```python
from build123d import *

# Parameters (mm, degrees)
F0_R     = 2.5
F1_DEPTH = 300


with BuildPart() as f1:
    # F0 (on Top) → F1 (new body)
    with BuildSketch(Plane.XY):
        with BuildLine():
            ThreePointArc((-10.36, 12.5), (-11.873209, 11.873209), (-12.5, 10.36))
            Line((-12.5, 10.36), (-12.5, 4.32))
            ThreePointArc((-12.5, 4.32), (-11.43, 3.25), (-10.36, 4.32))
            Line((-10.36, 4.32), (-10.36, 6.263583))
            ThreePointArc((-10.36, 6.263583), (-9.699471, 7.252134), (-8.533396, 7.020187))
            Line((-8.533396, 7.020187), (-4.363396, 2.850187))
            ThreePointArc((-4.363396, 2.850187), (-4.131449, 2.503054), (-4.05, 2.093583))
            Line((-4.05, 2.093583), (-4.05, 0))
            Line((-4.05, 0), (-4.05, -2.093583))
            ThreePointArc((-4.05, -2.093583), (-4.131449, -2.503054), (-4.363396, -2.850187))
            Line((-4.363396, -2.850187), (-8.533396, -7.020187))
            ThreePointArc((-8.533396, -7.020187), (-9.699471, -7.252134), (-10.36, -6.263583))
            Line((-10.36, -6.263583), (-10.36, -4.32))
            ThreePointArc((-10.36, -4.32), (-11.43, -3.25), (-12.5, -4.32))
            Line((-12.5, -4.32), (-12.5, -12.5))
            Line((-12.5, -12.5), (-12.5, -20.68))
            ThreePointArc((-12.5, -20.68), (-11.43, -21.75), (-10.36, -20.68))
            Line((-10.36, -20.68), (-10.36, -18.736417))
            ThreePointArc((-10.36, -18.736417), (-9.699471, -17.747866), (-8.533396, -17.979813))
            Line((-8.533396, -17.979813), (-4.363396, -22.149813))
            ThreePointArc((-4.363396, -22.149813), (-4.131449, -22.496946), (-4.05, -22.906417))
            Line((-4.05, -22.906417), (-4.05, -25))
            Line((-4.05, -25), (-4.05, -27.093583))
            ThreePointArc((-4.05, -27.093583), (-4.131449, -27.503054), (-4.363396, -27.850187))
            Line((-4.363396, -27.850187), (-8.533396, -32.020187))
            ThreePointArc((-8.533396, -32.020187), (-9.699471, -32.252134), (-10.36, -31.263583))
            Line((-10.36, -31.263583), (-10.36, -29.32))
            ThreePointArc((-10.36, -29.32), (-11.43, -28.25), (-12.5, -29.32))
            Line((-12.5, -29.32), (-12.5, -35.36))
            ThreePointArc((-12.5, -35.36), (-11.873209, -36.873209), (-10.36, -37.5))
            Line((-10.36, -37.5), (-4.32, -37.5))
            ThreePointArc((-4.32, -37.5), (-3.25, -36.43), (-4.32, -35.36))
            Line((-4.32, -35.36), (-6.263583, -35.36))
            ThreePointArc((-6.263583, -35.36), (-7.252134, -34.699471), (-7.020187, -33.533396))
            Line((-7.020187, -33.533396), (-3.310187, -29.823396))
            ThreePointArc((-3.310187, -29.823396), (-2.963054, -29.591449), (-2.553583, -29.51))
            Line((-2.553583, -29.51), (0, -29.51))
            Line((0, -29.51), (2.553583, -29.51))
            ThreePointArc((2.553583, -29.51), (2.963054, -29.591449), (3.310187, -29.823396))
            Line((3.310187, -29.823396), (7.020187, -33.533396))
            ThreePointArc((7.020187, -33.533396), (7.252134, -34.699471), (6.263583, -35.36))
            Line((6.263583, -35.36), (4.32, -35.36))
            ThreePointArc((4.32, -35.36), (3.25, -36.43), (4.32, -37.5))
            Line((4.32, -37.5), (10.36, -37.5))
            ThreePointArc((10.36, -37.5), (11.873209, -36.873209), (12.5, -35.36))
            Line((12.5, -35.36), (12.5, -29.32))
            ThreePointArc((12.5, -29.32), (11.43, -28.25), (10.36, -29.32))
            Line((10.36, -29.32), (10.36, -31.263583))
            ThreePointArc((10.36, -31.263583), (9.699471, -32.252134), (8.533396, -32.020187))
            Line((8.533396, -32.020187), (4.363396, -27.850187))
            ThreePointArc((4.363396, -27.850187), (4.131449, -27.503054), (4.05, -27.093583))
            Line((4.05, -27.093583), (4.05, -25))
            Line((4.05, -25), (4.05, -22.906417))
            ThreePointArc((4.05, -22.906417), (4.131449, -22.496946), (4.363396, -22.149813))
            Line((4.363396, -22.149813), (8.533396, -17.979813))
            ThreePointArc((8.533396, -17.979813), (9.699471, -17.747866), (10.36, -18.736417))
            Line((10.36, -18.736417), (10.36, -20.68))
            ThreePointArc((10.36, -20.68), (11.43, -21.75), (12.5, -20.68))
            Line((12.5, -20.68), (12.5, -12.5))
            Line((12.5, -12.5), (12.5, -4.32))
            ThreePointArc((12.5, -4.32), (11.43, -3.25), (10.36, -4.32))
            Line((10.36, -4.32), (10.36, -6.263583))
            ThreePointArc((10.36, -6.263583), (9.699471, -7.252134), (8.533396, -7.020187))
            Line((8.533396, -7.020187), (4.363396, -2.850187))
            ThreePointArc((4.363396, -2.850187), (4.131449, -2.503054), (4.05, -2.093583))
            Line((4.05, -2.093583), (4.05, 0))
            Line((4.05, 0), (4.05, 2.093583))
            ThreePointArc((4.05, 2.093583), (4.131449, 2.503054), (4.363396, 2.850187))
            Line((4.363396, 2.850187), (8.533396, 7.020187))
            ThreePointArc((8.533396, 7.020187), (9.699471, 7.252134), (10.36, 6.263583))
            Line((10.36, 6.263583), (10.36, 4.32))
            ThreePointArc((10.36, 4.32), (11.43, 3.25), (12.5, 4.32))
            Line((12.5, 4.32), (12.5, 10.36))
            ThreePointArc((12.5, 10.36), (11.873209, 11.873209), (10.36, 12.5))
            Line((10.36, 12.5), (4.32, 12.5))
            ThreePointArc((4.32, 12.5), (3.25, 11.43), (4.32, 10.36))
            Line((4.32, 10.36), (6.263583, 10.36))
            ThreePointArc((6.263583, 10.36), (7.252134, 9.699471), (7.020187, 8.533396))
            Line((7.020187, 8.533396), (3.310187, 4.823396))
            ThreePointArc((3.310187, 4.823396), (2.963054, 4.591449), (2.553583, 4.51))
            Line((2.553583, 4.51), (0, 4.51))
            Line((0, 4.51), (-2.553583, 4.51))
            ThreePointArc((-2.553583, 4.51), (-2.963054, 4.591449), (-3.310187, 4.823396))
            Line((-3.310187, 4.823396), (-7.020187, 8.533396))
            ThreePointArc((-7.020187, 8.533396), (-7.252134, 9.699471), (-6.263583, 10.36))
            Line((-6.263583, 10.36), (-4.32, 10.36))
            ThreePointArc((-4.32, 10.36), (-3.25, 11.43), (-4.32, 12.5))
            Line((-4.32, 12.5), (-10.36, 12.5))
        make_face()
        with Locations((0, -25)):
            Circle(F0_R, mode=Mode.SUBTRACT)
        with BuildLine():
            Line((-2.553583, -4.51), (0, -4.51))
            Line((0, -4.51), (2.553583, -4.51))
            ThreePointArc((2.553583, -4.51), (2.963054, -4.591449), (3.310187, -4.823396))
            Line((3.310187, -4.823396), (7.646979, -9.160187))
            ThreePointArc((7.646979, -9.160187), (7.994112, -9.392134), (8.403583, -9.473583))
            Line((8.403583, -9.473583), (9.29, -9.473583))
            ThreePointArc((9.29, -9.473583), (10.046604, -9.786979), (10.36, -10.543583))
            Line((10.36, -10.543583), (10.36, -12.5))
            Line((10.36, -12.5), (10.36, -14.456417))
            ThreePointArc((10.36, -14.456417), (10.046604, -15.213021), (9.29, -15.526417))
            Line((9.29, -15.526417), (8.403583, -15.526417))
            ThreePointArc((8.403583, -15.526417), (7.994112, -15.607866), (7.646979, -15.839813))
            Line((7.646979, -15.839813), (3.310187, -20.176604))
            ThreePointArc((3.310187, -20.176604), (2.963054, -20.408551), (2.553583, -20.49))
            Line((2.553583, -20.49), (0, -20.49))
            Line((0, -20.49), (-2.553583, -20.49))
            ThreePointArc((-2.553583, -20.49), (-2.963054, -20.408551), (-3.310187, -20.176604))
            Line((-3.310187, -20.176604), (-7.646979, -15.839813))
            ThreePointArc((-7.646979, -15.839813), (-7.994112, -15.607866), (-8.403583, -15.526417))
            Line((-8.403583, -15.526417), (-9.29, -15.526417))
            ThreePointArc((-9.29, -15.526417), (-10.046604, -15.213021), (-10.36, -14.456417))
            Line((-10.36, -14.456417), (-10.36, -12.5))
            Line((-10.36, -12.5), (-10.36, -10.543583))
            ThreePointArc((-10.36, -10.543583), (-10.046604, -9.786979), (-9.29, -9.473583))
            Line((-9.29, -9.473583), (-8.403583, -9.473583))
            ThreePointArc((-8.403583, -9.473583), (-7.994112, -9.392134), (-7.646979, -9.160187))
            Line((-7.646979, -9.160187), (-3.310187, -4.823396))
            ThreePointArc((-3.310187, -4.823396), (-2.963054, -4.591449), (-2.553583, -4.51))
        make_face(mode=Mode.SUBTRACT)
        Circle(F0_R, mode=Mode.SUBTRACT)
    extrude(amount=F1_DEPTH)


solid = f1.part
```
Work out the finished part from the listing and answer in its coordinate system (mm). A direction names the side the tool comes from. Round coordinates to 2 decimals unless told otherwise and drop trailing zeros. Write each loop counter-clockwise with the first axis right and the second up, starting at its lowest first coordinate (ties: lowest second). Pieces come first, ordered by that corner, then holes. Notation, with made-up numbers: (-27.5, -13) -> (-13.5, -13) arc R11 cw to (-13.5, -3) -> close; hole circle Ø6 at (28.5, -35.5). An arc over 180 degrees is marked (long way). Write each question's results on one line, items separated by ' | '.
1) Which of the six approach directions +Z, -Z, +X, -X, +Y, -Y give full straight-line access (tool end or side, diameter ignored) to faces 4 (the flat face through (0, -4.51, 148)), 5 (the flat face through (0, 4.51, 148)), 6 (the flat face through (-7, 12.5, 148))?
Findings:
face 4: +Z, -Z | face 5: +Z, -Z, +Y | face 6: +Z, -Z, +X, -X, +Y
2) Consider line 1 along Y through (x, z) = (0, 156); line 2 along Y through (x, z) = (-4.25, 77); line 3 along X through (y, z) = (-31, 169.5). Determine where each line is inside the solid, lowest interval first. Write a range as [from, to].
Findings:
line 1: y = [-29.51, -27.5], [-22.5, -20.49], [-4.51, -2.5], [2.5, 4.51] | line 2: y = [-37.5, -35.36], [-30.76, -27.72], [-22.28, -19.24], [-5.76, -2.72], [2.72, 5.76], [10.36, 12.5] | line 3: x = [-12.5, -10.36], [-7.51, -4.49], [4.49, 7.51], [10.36, 12.5]
3) The part is cut by section A-A (x = 0). Write down the section's boundary in (y, z), and give its area (3 significant figures).
Findings:
outline: (-29.51, 0) -> (-27.5, 0) -> (-27.5, 300) -> (-29.51, 300) -> close; (-22.5, 0) -> (-20.49, 0) -> (-20.49, 300) -> (-22.5, 300) -> close; (-4.51, 0) -> (-2.5, 0) -> (-2.5, 300) -> (-4.51, 300) -> close; (2.5, 0) -> (4.51, 0) -> (4.51, 300) -> (2.5, 300) -> close | area: 2,410 mm²
4) Flat-ended cylindrical pins translate along their axes: pin 1 (5 mm diameter, centred on y = -28, z = 129, fed in from +X); pin 2 (4 mm diameter, centred on x = 0, y = 0, fed in from -Z); pin 3 (4 mm diameter, centred on x = 0, z = 93.5, fed in from -Y); pin 4 (1 mm diameter, centred on x = -1.5, z = 44.5, fed in from +Y). Find the tip coordinate at first contact, or state that the pin passes through.
Findings:
pin 1: stops at x = 12.5 | pin 2: passes through | pin 3: stops at y = -29.51 | pin 4: stops at y = 4.51
5) For a pull along Y with two mould halves and no side action, classify faces 1 (the flat face through (7, 12.5, 148)), 2 (the flat face through (0, -20.49, 148)), 3 (the flat face through (0, -29.51, 148)) as +Y half, -Y half, draft (parallel to the pull), parting line (faces both ways), or undercut.
Findings:
face 1: +Y half | face 2: undercut | face 3: -Y half
6) The part is cut by section B-B (z = 91). State how many separate pieces and enclosed holes the cut face has, and give its area (3 significant figures).
Findings:
separate pieces: 1 | enclosed holes: 3 | area: 476 mm²
